The model under review builds one solid part; all positions refer to its coordinate system, in mm. Round coordinates to 2 decimals unless told otherwise and drop trailing zeros. Order: outer loops, then holes, each group sorted by start corner. A loop starts at its lowest first (then second) coordinate and runs counter-clockwise, first axis right, second up.
1) Consider section A-A (x = 3.5). Give the boundary of the cut face in (y, z), then the cut area to 3 significant figures.
2) Consider section B-B (y = -15). Give the boundary of the cut face in (x, z), then the cut area to 3 significant figures.
3) Mouldability with a two-part tool opening along X and no side actions: class faces 1 (the face through (-5.43, -16.9, 1.52)), 2 (the face through (-0.25, 16.18, 1.48)), 3 (the face through (5.4, 16.93, 1.52)) as pulls with the +X half, pulls with the -X half, needs draft (parallel to the pull), parting line crosses it, or undercut.
4) Consider section C-C (y = 15). Give the boundary of the cut face in (x, z).
5) Consider section D-D (z = 2.1). Give the boundary of the cut face in (x, y), then the cut area to 3 significant figures.
6) Clearance check with a flat-ended pin moving along its axis: P1, Ø2, axis at x = 0, y = -15, coming from the -Z side. State where the tip first meets the part, or that it passes through.
7) To check wall thickness, follow L1, parallel to Y at x = 3.5, z = 1.3; L2, parallel to Y at x = 0, z = 2.3; L3, parallel to Y at x = -1.5, z = 1.8. State the ranges of each line that lie inside material, in increasing order.
from build123d import *

# Parameters (mm, degrees)
ESQUISSE1_W             = 12
ESQUISSE1_H             = 35
ESQUISSE1_R             = 1.4
BOSS_EXTRU_1_DEPTH      = 3
ESQUISSE2_R             = 1.4
ENL_V_MAT_EXTRU_1_DEPTH = 4
CONG_1_R                = 2


with BuildPart() as part:
    # Esquisse1 → Boss.-Extru.1 (new body)
    with BuildSketch(Plane.XY):
        Rectangle(ESQUISSE1_W, ESQUISSE1_H)
        with Locations((-1, 15)):
            Circle(ESQUISSE1_R, mode=Mode.SUBTRACT)
        with Locations((0, -15)):
            Circle(ESQUISSE1_R, mode=Mode.SUBTRACT)
    extrude(amount=BOSS_EXTRU_1_DEPTH)

    # Esquisse2 → Enlèv. mat.-Extru.1 (cut, through all)
    with BuildSketch(Plane(origin=(0, 0, 0), x_dir=(-1, 0, 0), z_dir=(0, 0, -1))):
        with Locations((-3.5, 15)):
            Circle(ESQUISSE2_R)
    extrude(amount=-ENL_V_MAT_EXTRU_1_DEPTH, mode=Mode.SUBTRACT)

    # Congé1
    cong_1_edges = [part.edges().sort_by_distance(p)[0] for p in [
        (-6, 17.5, 1.5),
        (6, 17.5, 1.5),
        (6, -17.5, 1.5),
        (-6, -17.5, 1.5),
    ]]
    fillet(cong_1_edges, radius=CONG_1_R)


solid = part.part
Answer below:
1. outline: (-17.5, 0) - (13.6, 0) - (13.6, 3) - (-17.5, 3) - close; (16.4, 0) - (17.5, 0) - (17.5, 3) - (16.4, 3) - close
1. area: 96.6 mm2
2. outline: (-6, 0) - (-1.4, 0) - (-1.4, 3) - (-6, 3) - close; (1.4, 0) - (6, 0) - (6, 3) - (1.4, 3) - close
2. area: 27.6 mm2
3. face 1: pulls with the -X half
3. face 2: undercut
3. face 3: pulls with the +X half
4. outline: (-6, 0) - (-2.4, 0) - (-2.4, 3) - (-6, 3) - close; (0.4, 0) - (2.1, 0) - (2.1, 3) - (0.4, 3) - close; (4.9, 0) - (6, 0) - (6, 3) - (4.9, 3) - close
5. outline: (-6, -15.5) arc R2 ccw to (-4, -17.5) - (4, -17.5) arc R2 ccw to (6, -15.5) - (6, 15.5) arc R2 ccw to (4, 17.5) - (-4, 17.5) arc R2 ccw to (-6, 15.5) - close; hole circle Ø2.8 at (-1, 15); hole circle Ø2.8 at (0, -15); hole circle Ø2.8 at (3.5, 15)
5. area: 398 mm2
6. P1: passes through
7. L1: y = -17.5 to 13.6, 16.4 to 17.5
7. L2: y = -17.5 to -16.4, -13.6 to 14.02, 15.98 to 17.5
7. L3: y = -17.5 to 13.69, 16.31 to 17.5
